Source: CAD feature listing. Evaluate the final solid. Frame: model axes, mm. Coordinates: 2 decimals unless noted, no trailing zeros. Order: outer loops, then holes, each group sorted by start corner. A loop starts at its lowest first (then second) coordinate and runs counter-clockwise, first axis right, second up.
```python
from build123d import *

# Parameters (mm, degrees)
SKETCH4_R = 0.508


with BuildPart() as part:
    # Sweep1: sweep along a curve in space
    with BuildLine() as sweep1_path:
        Line((17.526, 6.604, -4.102670361), (17.526, 1.27, -4.102670361))
        ThreePointArc((17.526, 1.27, -4.102670361), (17.191671635, 0.371974388, -4.2657332), (16.384531561, 0, -4.659401718))
        Line((16.384531561, 0, -4.659401718), (5.97077017, 0, -9.738532518))
        ThreePointArc((5.97077017, 0, -9.738532518), (4.519904893, 0, -9.865466782), (3.356766269, 0, -8.988978961))
        Line((3.356766269, 0, -8.988978961), (0.971149403, 0, -5.171193917))
        ThreePointArc((0.971149403, 0, -5.171193917), (0.890159133, 0, -2.078300277), (3.556, 0, -0.508))
        Line((3.556, 0, -0.508), (19.003402457, 0, -0.508))
        ThreePointArc((19.003402457, 0, -0.508), (19.861402021, 0, -0.841657782), (20.268569724, 0, -1.667312207))
        Line((20.268569724, 0, -1.667312207), (20.829933093, 0, -8.083724883))
    # Sketch4 → Sweep1 (sweep)
    with BuildSketch(Plane(origin=(0, 6.604, 0), x_dir=(1, 0, 0), z_dir=(0, 1, 0))):
        with Locations((17.526, 4.102670361)):
            Circle(SKETCH4_R)
    sweep(path=sweep1_path.line)


solid = part.part
```
1. Pin query (flat end, axial travel): P1, Ø1, axis at x = 19, z = -3, coming from the -Y side; P2, Ø3, axis at x = 17, z = -2, coming from the +Y side. Return the tip coordinate at first contact, or that it passes through.
Findings:
P1: passes through
P2: stops at y = 0.51
2. Draft query along Z for faces 1 (the face through (17.15, 3.9, -3.76)), 2 (the face through (20.823, 0.007, -8.084)), 3 (the face through (17.5, 6.604, -4.1)), 4 (the face through (11.39, -0.16, -0.99)). Return one class per face: released by +Z, released by -Z, zero draft, split by the parting line, or undercut.
Findings:
face 1: split by the parting line
face 2: released by -Z
face 3: zero draft
face 4: undercut
3. Ray query, line 1 (Z direction, x = 17.75, y = 0); line 2 (Y direction, x = 13, z = -6.75); line 3 (Y direction, x = 11, z = -7.25). Return the intervals inside material, ascending.
Findings:
line 1: z = -1.02 to 0
line 2: y = -0.32 to 0.32
line 3: y = -0.51 to 0.51
4. Section query B-B on z = -7.25. Count the separate pieces of the cut face and the enclosed holes in it, plus the area to 3 significant figures.
Findings:
separate pieces: 3
enclosed holes: 0
area: 3.62 mm2
5. Section query A-A on y = 1.5. Return loops of the section in (x, z), plus the area to 3 significant figures.
Findings:
outline: circle Ø1.02 at (17.53, -4.1)
area: 0.811 mm2
